Geometry: final body of the model. Coordinates: model frame, mm. Face numbers are marked on the shaded views. A direction names the side the tool comes from. Give positions to 0.01 mm unless a question says otherwise; leave off trailing zeros. Loops run counter-clockwise (first coordinate to the right, second up) from the corner with the lowest first, then second, coordinate; pieces in that order, holes last. Notation, with made-up numbers: M -14.75,26 L 7.25,26 A37 ccw 7.25,63 Z; hole C 5.5,20 d7. An arc over 180 degrees is marked long. Put each result on its own line as item: value.
```python
from build123d import *

# Parameters (mm, degrees)
F0_R     = 11.25
F1_DEPTH = 25
F3_DEPTH = 25
F4_R     = 3.25
F5_DEPTH = 4
F6_W     = 12
F6_H     = 4.5
F7_DEPTH = 19
F8_R     = 3
F9_DEPTH = 12
F10_R    = 5
F11_R    = 5
F12_R    = 1.99999


# Not quite as in the source:
# - a fillet or chamfer is up to 0.001 mm smaller than in the source, because OpenCascade refuses the exact size


with BuildPart() as f1:
    # F0 (on Top) → F1 (new body)
    with BuildSketch(Plane.XY):
        with BuildLine():
            Line((-81.25, 25.15), (-81.25, -25.15))
            Line((-81.25, -25.15), (-111.25, -25.15))
            Line((-111.25, -25.15), (-111.25, -29.15))
            Line((-111.25, -29.15), (-77.25, -29.15))
            Line((-77.25, -29.15), (-77.25, -3))
            Line((-77.25, -3), (-14.9520065543, -3))
            ThreePointArc((-14.9520065543, -3), (-13.8519724825, -6.3785075325), (-12, -9.4107651124))
            Line((-12, -9.4107651124), (-12, -12.3110722522))
            Line((-12, -12.3110722522), (-12, -21.25))
            Line((-12, -21.25), (-9, -21.25))
            Line((-9, -21.25), (9, -21.25))
            Line((9, -21.25), (12, -21.25))
            Line((12, -21.25), (12, -12.3110722522))
            Line((12, -12.3110722522), (12, -9.4107651124))
            ThreePointArc((12, -9.4107651124), (6.3785075325, 13.8519724825), (-14.9520065543, 3))
            Line((-14.9520065543, 3), (-77.25, 3))
            Line((-77.25, 3), (-77.25, 29.15))
            Line((-77.25, 29.15), (-111.25, 29.15))
            Line((-111.25, 29.15), (-111.25, 25.15))
            Line((-111.25, 25.15), (-81.25, 25.15))
        make_face()
        Circle(F0_R, mode=Mode.SUBTRACT)
    extrude(amount=F1_DEPTH)

    # F2 (on face) → F3 (join)
    with BuildSketch(Plane.XY.offset(25)):
        Polygon((-77.25, 3), (-77.25, 29.15), (-81.25, 29.15), (-81.25, 25.15), (-81.25, -25.15), (-81.25, -29.15), (-77.25, -29.15), (-77.25, -3), align=None)
    extrude(amount=F3_DEPTH)

    # F4 (on face) → F5 (cut)
    with BuildSketch(Plane.YZ.offset(-77.25)):
        with Locations((0, 37.5)):
            Circle(F4_R)
    extrude(amount=-F5_DEPTH, mode=Mode.SUBTRACT)

    # F6 (on face) → F7 (cut)
    with BuildSketch(Plane.XY.offset(25)):
        with Locations((0, -15)):
            Rectangle(F6_W, F6_H)
    extrude(amount=-F7_DEPTH, mode=Mode.SUBTRACT)

    # F8 (on face) → F9 (cut)
    with BuildSketch(Plane.XZ.offset(21.25)):
        with Locations((0, 12.5)):
            Circle(F8_R)
    extrude(amount=-F9_DEPTH, mode=Mode.SUBTRACT)

    # F10
    f10_edges = [f1.edges().sort_by_distance(p)[0] for p in [
        (12, -21.25, 12.5),
        (-12, -21.25, 12.5),
        (-77.25, -3, 12.5),
        (-77.25, 3, 12.5),
    ]]
    fillet(f10_edges, radius=F10_R)

    # F11
    f11_edges = [f1.edges().sort_by_distance(p)[0] for p in [
        (-14.952007, 3, 12.5),
        (-14.952007, -3, 12.5),
        (-77.25, 0, 25),
    ]]
    fillet(f11_edges, radius=F11_R)

    # F12 (radius 2 in the source; OpenCascade refuses exactly that, so slightly less here)
    f12_edges = [f1.edges().sort_by_distance(p)[0] for p in [
        (-111.25, 29.15, 12.5),
        (-111.25, -25.15, 12.5),
        (-111.25, -29.15, 12.5),
        (-111.25, 25.15, 12.5),
        (-77.25, 29.15, 25),
        (-81.25, 29.15, 37.5),
        (-77.25, -29.15, 25),
        (-81.25, -29.15, 37.5),
    ]]
    fillet(f12_edges, radius=F12_R)


solid = f1.part
```
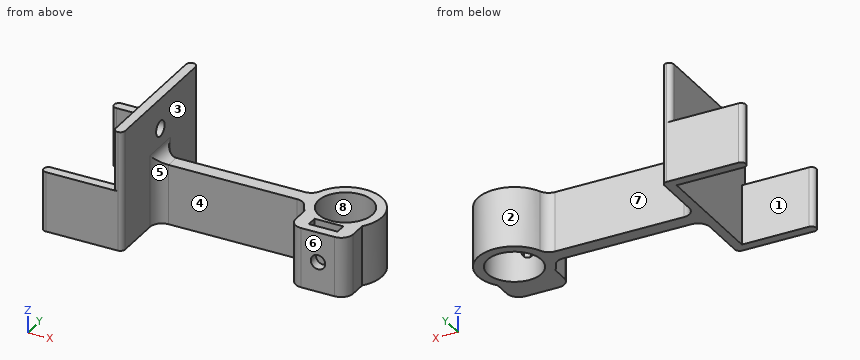
Item 1: Section D-D on y = 21.5. Output: boundary loops of the cut face in (x, z), then the cut area to 3 significant figures.
Output values:
outline: M -81.25,0 L -77.25,0 L -77.25,50 L -81.25,50 Z
area: 200 mm²
Item 2: Line query: probe 1 along X at (y, z) = (-11.3, 12.5); probe 2 along Z at (x, y) = (0, -19.5); probe 3 along X at (y, z) = (-7, 16.5). Output: solid intervals per line, ascending. Write a range as [from, to].
Output values:
probe 1: [-81.25, -77.25], [-12, -3], [3, 12]
probe 2: [0, 9.5], [15.5, 25]
probe 3: [-81.25, -77.15], [-13.55, -8.81], [8.81, 13.55]
Item 3: Set-up query: the marked faces 5, 6, 7 and 8. Return all of +Z, -Z, +X, -X, +Y, -Y with unobstructed straight access to the full face (end or side cutting, diameter ignored); none if empty.
Output values:
face 5: +Z, -Z, -Y
face 6: +Z, -Z, +X, -Y
face 7: +Z, -Z, +Y
face 8: +Z, -Z
Item 4: Section A-A on x = 0. Output: boundary loops of the cut face in (y, z), then the cut area to 4 significant figures.
Output values:
outline: M -21.25,0 L -11.25,0 L -11.25,9.5 L -12.75,9.5 L -12.75,6 L -17.25,6 L -17.25,9.5 L -21.25,9.5 Z; M -21.25,15.5 L -17.25,15.5 L -17.25,25 L -21.25,25 Z; M -12.75,15.5 L -11.25,15.5 L -11.25,25 L -12.75,25 Z; M 11.25,0 L 15.25,0 L 15.25,25 L 11.25,25 Z
area: 231.5 mm²
Item 5: Mould query, pull axis Y, two halves, no side actions, for the marked faces 1, 2, 3 and 4. Classes: pulls with the +Y half, pulls with the -Y half, needs draft (parallel to the pull), parting line crosses it, or undercut.
Output values:
face 1: undercut
face 2: parting line crosses it
face 3: needs draft
face 4: pulls with the -Y half
Item 6: Pin query (flat end, axial travel): pin 1 Ø2 at (y, z) = (4, 37) entering from +X; pin 2 Ø4 at (y, z) = (0, 37.5) entering from -X; pin 3 Ø1.3 at (x, y) = (1.5, -15.5) entering from +Z; pin 4 Ø6 at (x, z) = (0.5, 17.5) entering from +Y. Return the tip coordinate at first contact, or that it passes through.
Output values:
pin 1: x = -77.25
pin 2: through
pin 3: z = 6
pin 4: y = 15.25
Item 7: Section C-C on y = 0. Output: boundary loops of the cut face in (x, z).
Output values:
outline: M -81.25,0 L -11.25,0 L -11.25,25 L -72.25,25 A5 cw -77.25,30 L -77.25,34.25 L -81.25,34.25 Z; M -81.25,40.75 L -77.25,40.75 L -77.25,50 L -81.25,50 Z; M 11.25,0 L 15.25,0 L 15.25,25 L 11.25,25 Z
